Verification items for the finished model (mm, model axes). Face numbers are marked on the shaded views. Give positions to 0.01 mm unless a question says otherwise; leave off trailing zeros. Loops run counter-clockwise (first coordinate to the right, second up) from the corner with the lowest first, then second, coordinate; pieces in that order, holes last. Notation, with made-up numbers: (34.5, 11) - (60.5, 11) arc R7 ccw to (60.5, 18) - close; hole circle Ø3 at (-4.5, 25.25). An arc over 180 degrees is marked (long way). Answer in a Markdown table with one row per item.
```python
from build123d import *

# Parameters (mm, degrees)
SKETCH1_R               = 10
SKETCH1_R_2             = 9
BOSS_EXTRUDE1_DEPTH     = 170
BOSS_EXTRUDE2_START     = -10
BOSS_EXTRUDE2_DEPTH     = 10
CUT_EXTRUDE1_DEPTH      = 171.862672505
CUT_EXTRUDE1_DEPTH_BACK = 171.862672505
SKETCH3_R               = 2.5


with BuildPart() as part:
    # Sketch1 → Boss-Extrude1 (new body)
    with BuildSketch(Plane.XY):
        Circle(SKETCH1_R)
        Circle(SKETCH1_R_2, mode=Mode.SUBTRACT)
    extrude(amount=BOSS_EXTRUDE1_DEPTH)

    # Sketch2 → Boss-Extrude2 (add)
    with BuildSketch(Plane.XY.offset(170).offset(BOSS_EXTRUDE2_START)):
        with BuildLine():
            Line((-9.43028555, 4.5), (-8.93028555, 4.5))
            ThreePointArc((-8.93028555, 4.5), (-10, 0), (-8.93028555, -4.5))
            Line((-8.93028555, -4.5), (-9.43028555, -4.5))
            ThreePointArc((-9.43028555, -4.5), (-13.93028555, 0), (-9.43028555, 4.5))
        make_face()
        with BuildLine():
            Line((8.93028555, 4.5), (9.43028555, 4.5))
            ThreePointArc((9.43028555, 4.5), (13.93028555, 0), (9.43028555, -4.5))
            Line((9.43028555, -4.5), (8.93028555, -4.5))
            ThreePointArc((8.93028555, -4.5), (10, 0), (8.93028555, 4.5))
        make_face()
    extrude(amount=BOSS_EXTRUDE2_DEPTH)

    # Sketch3 → Cut-Extrude1 (cut, two sides: drawn at the far end of the back side and taken through both)
    with BuildSketch(Plane(origin=(0, 0, 0), x_dir=(1, 0, 0), z_dir=(0, 1, 0)).offset(-CUT_EXTRUDE1_DEPTH_BACK)):
        with Locations(Location((0, -10, 0), (0, 0, 270))):
            Circle(SKETCH3_R)
    extrude(amount=CUT_EXTRUDE1_DEPTH + CUT_EXTRUDE1_DEPTH_BACK, mode=Mode.SUBTRACT)


solid = part.part
```
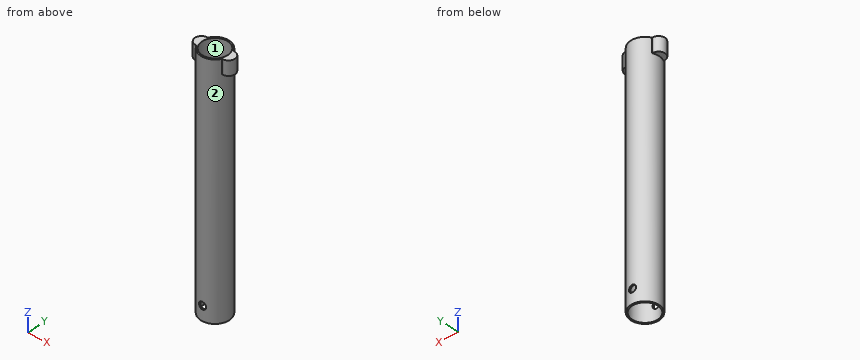
Q1. Go/stop test with flat-tipped pins: P1, Ø1, axis at x = 2.5, y = 7.5, coming from the -Z side; P2, Ø5, axis at y = -7, z = 141, coming from the -X side; P3, Ø10, axis at y = 3.5, z = 104.5, coming from the +X side; P4, Ø1.5, axis at x = 12.5, y = 1.5, coming from the -Z side. Record where each tip stops, or that it passes through.
Completed:
| item | result |
|---|---|
| P1 | through |
| P2 | x = -8.93 |
| P3 | x = 10 |
| P4 | z = 160 |
Q2. Sectioned sample at D-D (z = 63). Record the cut outline in (x, y), and give its area (3 significant figures).
Completed:
| item | result |
|---|---|
| outline | circle Ø20 at (0, 0); hole circle Ø18 at (0, 0) |
| area | 59.7 mm^2 |
Q3. Sectioned sample at B-B (x = 0). Record the cut outline in (y, z), and give its area (3 significant figures).
Completed:
| item | result |
|---|---|
| outline | (-10, 0) - (-9, 0) - (-9, 7.5) - (-10, 7.5) - close; (-10, 12.5) - (-9, 12.5) - (-9, 170) - (-10, 170) - close; (9, 0) - (10, 0) - (10, 7.5) - (9, 7.5) - close; (9, 12.5) - (10, 12.5) - (10, 170) - (9, 170) - close |
| area | 330 mm^2 |
Q4. Sectioned sample at C-C (z = 10). Record the cut outline in (x, y), and give its area (3 significant figures).
Completed:
| item | result |
|---|---|
| outline | (-2.5, -9.68) - (-2.5, -8.65) arc R9 cw to (-2.5, 8.65) - (-2.5, 9.68) arc R10 ccw to start; (2.5, -9.68) arc R10 ccw to (2.5, 9.68) - (2.5, 8.65) arc R9 cw to (2.5, -8.65) - close |
| area | 49.6 mm^2 |
Q5. Sectioned sample at A-A (y = 0). Record the cut outline in (x, z), and give its area (3 significant figures).
Completed:
| item | result |
|---|---|
| outline | (-13.93, 160) - (-10, 160) - (-10, 0) - (-9, 0) - (-9, 170) - (-13.93, 170) - close; (9, 0) - (10, 0) - (10, 160) - (13.93, 160) - (13.93, 170) - (9, 170) - close |
| area | 419 mm^2 |
Q6. Thickness scan on line 1 (Z direction, x = 0, y = -9.3); line 2 (Y direction, x = 0, z = 77); line 3 (Y direction, x = -8.25, z = 124). Record the ranges inside material, lowest first.
Completed:
| item | result |
|---|---|
| line 1 | 0 to 7.5, 12.5 to 170 |
| line 2 | -10 to -9, 9 to 10 |
| line 3 | -5.65 to -3.6, 3.6 to 5.65 |
Q7. Draft check along Y on the marked faces 1 and 2. Enter one of: +Y half, -Y half, draft (parallel to the pull), parting line (faces both ways), or undercut.
Completed:
| item | result |
|---|---|
| face 1 | undercut |
| face 2 | parting line |
